Source: CAD feature listing. Evaluate the final solid. Frame: model axes, mm. Face numbers are marked on the shaded views. Round coordinates to 2 decimals unless told otherwise and drop trailing zeros. Write each loop counter-clockwise with the first axis right and the second up, starting at its lowest first coordinate (ties: lowest second). Pieces come first, ordered by that corner, then holes. Notation, with made-up numbers: M 65,47 L 81,47 A5 ccw 81,55 Z; hole C 39.25,-20 d11. An arc over 180 degrees is marked long. Put each result on its own line as item: value. Start each with the question number.
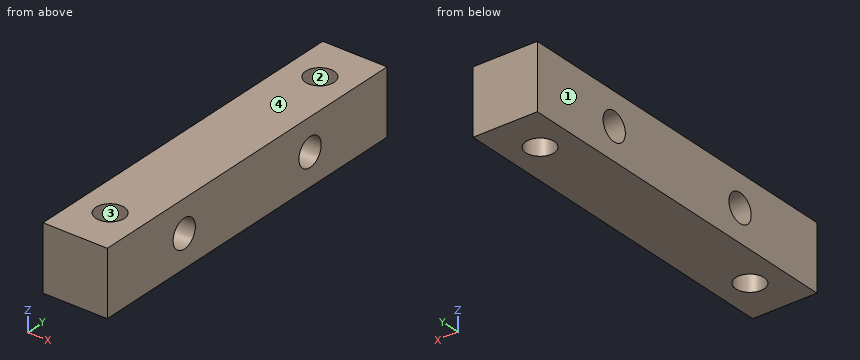
```python
from build123d import *

# Parameters (mm, degrees)
SKETCH1_W                  = 9.144
SKETCH1_H                  = 9.144
BOSS_EXTRUDE1_DEPTH        = 50.8
TAP_DRILL_FOR_10_32_TAP1_D = 4.0386
TAP_DRILL_FOR_10_32_TAP2_D = 4.0386


with BuildPart() as part:
    # Sketch1 → Boss-Extrude1 (new body)
    with BuildSketch(Plane(origin=(0, 0, 0), x_dir=(1, 0, 0), z_dir=(0, 1, 0))):
        Rectangle(SKETCH1_W, SKETCH1_H)
    extrude(amount=BOSS_EXTRUDE1_DEPTH)

    # Tap Drill for #10-32 Tap1 (through all)
    with Locations(Plane.XY.offset(4.572)):
        with Locations((0, 44.45), (0, 6.35)):
            Hole(TAP_DRILL_FOR_10_32_TAP1_D / 2)

    # Tap Drill for #10-32 Tap2 (through all)
    with Locations(Plane(origin=(4.572, 0, 0), x_dir=(0, 0, -1), z_dir=(1, 0, 0))):
        with Locations((0, 36.83), (0, 13.97)):
            Hole(TAP_DRILL_FOR_10_32_TAP2_D / 2)


solid = part.part
```
(1) Contact query for a flat-ended pin moving along its axis: P1, Ø3.5, axis at x = 0, y = 44.45, coming from the +Z side. Output: stop coordinate, or through.
(2) Ray query, line 1 along Z through (x, y) = (-2.75, 37); line 2 along Y through (x, z) = (0, -1.5); line 3 along Y through (x, z) = (-3.25, -1). Return the intervals inside material, ascending.
(3) Section query B-B (x = 0). Return loops of the section in (y, z).
(4) Section query D-D (z = 3.5). Return loops of the section in (x, y), and give its area (3 significant figures).
(5) Section query A-A (z = 0). Return loops of the section in (x, y).
(6) Section query C-C (y = 36.83). Return loops of the section in (x, z).
(7) Pull-direction query (X, two-part tool) for the marked faces 1, 2, 3 and 4; classes: +X half, -X half, draft (parallel to the pull), parting line (faces both ways), or undercut.
Entries:
1. P1: through
2. line 1: -4.57 to -2.01, 2.01 to 4.57
2. line 2: 0 to 4.33, 8.37 to 12.62, 15.32 to 35.48, 38.18 to 42.43, 46.47 to 50.8
2. line 3: 0 to 12.22, 15.72 to 35.08, 38.58 to 50.8
3. outline: M 0,-4.57 L 4.33,-4.57 L 4.33,4.57 L 0,4.57 Z; M 8.37,-4.57 L 42.43,-4.57 L 42.43,4.57 L 8.37,4.57 Z; M 46.47,-4.57 L 50.8,-4.57 L 50.8,4.57 L 46.47,4.57 Z; hole C 13.97,0 d4.04; hole C 36.83,0 d4.04
4. outline: M -4.57,0 L 4.57,0 L 4.57,50.8 L -4.57,50.8 Z; hole C 0,6.35 d4.04; hole C 0,44.45 d4.04
4. area: 439 mm2
5. outline: M -4.57,0 L 4.57,0 L 4.57,11.95 L -4.57,11.95 Z; M -4.57,15.99 L 4.57,15.99 L 4.57,34.81 L -4.57,34.81 Z; M -4.57,38.85 L 4.57,38.85 L 4.57,50.8 L -4.57,50.8 Z; hole C 0,6.35 d4.04; hole C 0,44.45 d4.04
6. outline: M -4.57,-4.57 L 4.57,-4.57 L 4.57,-2.02 L -4.57,-2.02 Z; M -4.57,2.02 L 4.57,2.02 L 4.57,4.57 L -4.57,4.57 Z
7. face 1: -X half
7. face 2: undercut
7. face 3: undercut
7. face 4: draft
